Source: CAD feature listing. Evaluate the final solid. Frame: model axes, mm. Face numbers are marked on the shaded views. A direction names the side the tool comes from. Give positions to 0.01 mm unless a question says otherwise; leave off trailing zeros. Loops run counter-clockwise (first coordinate to the right, second up) from the corner with the lowest first, then second, coordinate; pieces in that order, holes last. Notation, with made-up numbers: (-39, 30) - (-20, 30) arc R16 cw to (-20, 42) - close; hole circle Ø8 at (-17.75, 21). An arc over 180 degrees is marked (long way). Put each result on its own line as item: value.
```python
from build123d import *

# Parameters (mm, degrees)
F1_DEPTH = 10
F3_DEPTH = 1.6
F5_DEPTH = 24
F7_DEPTH = 90
F9_DEPTH = 90
F10_D    = 5


with BuildPart() as f1:
    # F0 (on Front) → F1 (new body)
    with BuildSketch(Plane.XZ):
        with BuildLine():
            ThreePointArc((0, 4), (1.1715728753, 1.1715728753), (4, 0))
            Line((4, 0), (56, 0))
            ThreePointArc((56, 0), (58.8284271247, 1.1715728753), (60, 4))
            Line((60, 4), (60, 56))
            ThreePointArc((60, 56), (58.8284271247, 58.8284271247), (56, 60))
            Line((56, 60), (4, 60))
            ThreePointArc((4, 60), (1.1715728753, 58.8284271247), (0, 56))
            Line((0, 56), (0, 4))
        make_face()
    extrude(amount=-F1_DEPTH)

    # F2 (on face) → F3 (join)
    with BuildSketch(Plane.XZ):
        with BuildLine():
            ThreePointArc((49.05, 30), (43.4703841816, 43.4703841816), (30, 49.05))
            Line((30, 49.05), (30, 10.95))
            ThreePointArc((30, 10.95), (43.4703841816, 16.5296158184), (49.05, 30))
        make_face()
        with BuildLine():
            Line((30, 10.95), (30, 49.05))
            ThreePointArc((30, 49.05), (10.95, 30), (30, 10.95))
        make_face()
    extrude(amount=F3_DEPTH)

    # F4 (on face) → F5 (join)
    with BuildSketch(Plane.XZ):
        with BuildLine():
            ThreePointArc((34.7625, 30), (33.3675960454, 33.3675960454), (30, 34.7625))
            Line((30, 34.7625), (30, 25.2375))
            ThreePointArc((30, 25.2375), (33.3675960454, 26.6324039546), (34.7625, 30))
        make_face()
        with BuildLine():
            Line((30, 25.2375), (30, 34.7625))
            ThreePointArc((30, 34.7625), (25.2375, 30), (30, 25.2375))
        make_face()
    extrude(amount=F5_DEPTH)

    # F7 (add): a face of the model
    f7_faces = [f1.faces().sort_by_distance(p)[0] for p in [
        (30, 10, 30),
    ]]
    extrude(f7_faces, amount=F7_DEPTH)

    # F8 (on face) → F9 (cut)
    with BuildSketch(Plane(origin=(0, 100, 0), x_dir=(-1, 0, 0), z_dir=(0, 1, 0))):
        with BuildLine():
            Line((-60, 50), (-54, 50))
            ThreePointArc((-54, 50), (-51.1715728753, 51.1715728753), (-50, 54))
            Line((-50, 54), (-50, 60))
            Line((-50, 60), (-60, 60))
            Line((-60, 60), (-60, 50))
        make_face()
        with BuildLine():
            ThreePointArc((-10, 54), (-8.8284271247, 51.1715728753), (-6, 50))
            Line((-6, 50), (0, 50))
            Line((0, 50), (0, 60))
            Line((0, 60), (-10, 60))
            Line((-10, 60), (-10, 54))
        make_face()
        with BuildLine():
            ThreePointArc((-50, 6), (-51.1715728753, 8.8284271247), (-54, 10))
            Line((-54, 10), (-60, 10))
            Line((-60, 10), (-60, 0))
            Line((-60, 0), (-50, 0))
            Line((-50, 0), (-50, 6))
        make_face()
        with BuildLine():
            Line((0, 10), (-6, 10))
            ThreePointArc((-6, 10), (-8.8284271247, 8.8284271247), (-10, 6))
            Line((-10, 6), (-10, 0))
            Line((-10, 0), (0, 0))
            Line((0, 0), (0, 10))
        make_face()
    extrude(amount=-F9_DEPTH, mode=Mode.SUBTRACT)

    # F10 (through all)
    with Locations(Plane.XZ):
        with Locations((6.43, 53.57), (53.57, 53.57), (53.57, 6.43), (6.43, 6.43)):
            Hole(F10_D / 2)


solid = f1.part
```
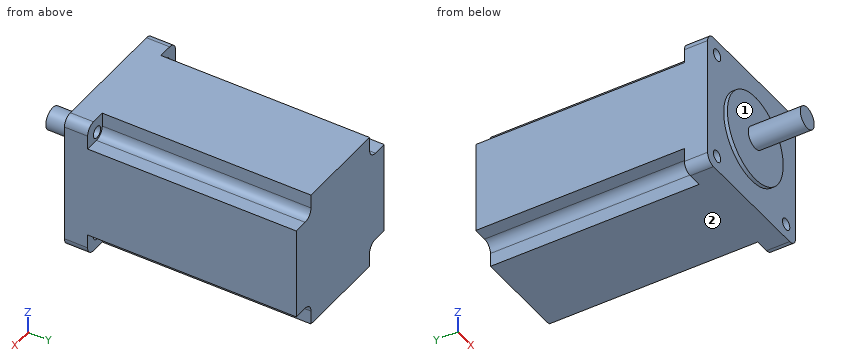
1) Section query A-A, the plane x = 30. Output: boundary loops of the cut face in (y, z), plus the area to 3 significant figures.
Check result:
outline: (-24, 25.24) - (-1.6, 25.24) - (-1.6, 10.95) - (0, 10.95) - (0, 0) - (100, 0) - (100, 60) - (0, 60) - (0, 49.05) - (-1.6, 49.05) - (-1.6, 34.76) - (-24, 34.76) - close
area: 6,270 mm²
2) Section query C-C, the plane y = 55. Output: boundary loops of the cut face in (x, z).
Check result:
outline: (0, 10) - (6, 10) arc R4 cw to (10, 6) - (10, 0) - (50, 0) - (50, 6) arc R4 cw to (54, 10) - (60, 10) - (60, 50) - (54, 50) arc R4 cw to (50, 54) - (50, 60) - (10, 60) - (10, 54) arc R4 cw to (6, 50) - (0, 50) - close
3) Access query for the marked faces 1 and 2. Directions: +Z, -Z, +X, -X, +Y, -Y. A direction counts if a zero-diameter tool reaches every point of the face in a straight line with its end or side. Return the directions, or none.
Check result:
face 1: -Y
face 2: -Z, +X, -X, +Y, -Y
4) Section query B-B, the plane z = 30. Output: boundary loops of the cut face in (x, y), plus the area to 3 significant figures.
Check result:
outline: (0, 0) - (10.95, 0) - (10.95, -1.6) - (25.24, -1.6) - (25.24, -24) - (34.76, -24) - (34.76, -1.6) - (49.05, -1.6) - (49.05, 0) - (60, 0) - (60, 100) - (0, 100) - close
area: 6,270 mm²
5) Section query D-D, the plane x = 36.5. Output: boundary loops of the cut face in (y, z), plus the area to 3 significant figures.
Check result:
outline: (-1.6, 12.09) - (0, 12.09) - (0, 0) - (100, 0) - (100, 60) - (0, 60) - (0, 47.91) - (-1.6, 47.91) - close
area: 6,060 mm²
6) Material intervals for line 1 along Z through (x, y) = (53.57, 3.5); line 2 along X through (y, z) = (8, 53), sorted ascending. Write a range as [from, to].
Check result:
line 1: [0, 3.93], [8.93, 51.07], [56.07, 60]
line 2: [0, 4], [8.86, 51.14], [56, 60]
7) Pin query (flat end, axial travel): P1, Ø5, axis at x = 57, y = 44.5, coming from the -Z side; P2, Ø6.5, axis at x = 6.43, z = 53.57, coming from the +Y side; P3, Ø12, axis at x = 11, z = 11.5, coming from the -Y side. Return the tip coordinate at first contact, or that it passes through.
Check result:
P1: z = 10
P2: y = 10
P3: y = 0
